Autodesk Inventor part; units mm, degrees
ref_plane "YZ Plane" through (0, 0, 0) normal (1, 0, 0) x (0, 1, 0)
ref_plane "XZ Plane" through (0, 0, 0) normal (0, 1, 0) x (-1, 0, 0)
ref_plane "XY Plane" through (0, 0, 0) normal (0, 0, 1) x (1, 0, 0)
sketch "Sketch1" plane through (0, 0, 0) normal (0, 1, 0) x (-1, 0, 0)
  line L0 (0, 0) -> (0, -14)
  circle A0 centre (0, -7) radius 8.25
  circle A1 centre (0, -7) radius 10.5
  dimension "d0" = 14
  dimension "d1" = 16.5
  dimension "d2" = 21
extrude "Extrusion1" add sketch "Sketch1" along normal blind 6
sketch "Sketch2" plane through (0, 6, -7) normal (0, 1, 0) x (1, 0, 0)
  line L0 (10.5, -10.5) -> (-10.5, -10.5)
  line L1 (-10.5, -10.5) -> (-10.5, 10.5)
  line L2 (-10.5, 10.5) -> (10.5, 10.5)
  line L3 (10.5, 10.5) -> (10.5, -10.5)
  line L4 (10.5, -10.5) -> (-10.5, 10.5) construction
  line L5 (-10.5, -10.5) -> (10.5, 10.5) construction
  circle A0 centre (0, 0) radius 10.5
  point P0 (0, -7)
extrude "Extrusion2" add sketch "Sketch2" against normal blind 6 contours L0 A0 L3 | L0 L1 A0 | A0 L2 L3 | L1 L2 A0
sketch "Sketch4" plane through (0, 6, 0) normal (0, 1, 0) x (1, 0, 0)
  circle A0 centre (0, 7) radius 8.25
  line L0 (0, 7) -> (0, -0.25)
  line L1 (0, -0.25) -> (-3.937, -0.25)
  line L2 (3.937, -0.25) -> (-3.937, -0.25)
  point P0 (0, 0)
  dimension "d14" = 7.25
extrude "Extrusion4" add sketch "Sketch4" against normal blind 6 contours L1 L2 A0 picked at (1.9893, -0.4987)
pattern_circular "Circular Pattern2" count 6 over 360 about axis through (0, 0, -7) along (0, 1, 0) of "Extrusion4"
sketch "Sketch5" plane through (0, 6, 0) normal (0, 1, 0) x (1, 0, 0)
  line L0 (-4.3102, -0.0345) -> (-8.2472, 6.7845)
  line L1 (-6.2787, 3.375) -> (6.2787, 10.625)
  line L2 (4.3102, 14.0345) -> (8.2472, 7.2155)
  line L3 (8.2472, 6.7845) -> (4.3102, -0.0345)
  line L4 (6.2787, 3.375) -> (-6.2787, 10.625)
  line L5 (-4.3102, 14.0345) -> (-8.2472, 7.2155)
  line L6 (3.937, 14.25) -> (-3.937, 14.25)
  line L7 (0, 14.25) -> (0, -0.25)
  line L8 (3.937, -0.25) -> (-3.937, -0.25)
  circle A0 centre (0, 7) radius 9.75
  line L9 (12.5, 19.5) -> (-12.5, 19.5)
  line L10 (-12.5, 19.5) -> (-12.5, -5.5)
  line L11 (-12.5, -5.5) -> (12.5, -5.5)
  line L12 (12.5, -5.5) -> (12.5, 19.5)
  line L13 (12.5, 19.5) -> (-12.5, -5.5) construction
  line L14 (-12.5, 19.5) -> (12.5, -5.5) construction
  point P0 (0, 0)
  dimension "d20" = 19.5
  dimension "d21" = 25
  dimension "d22" = 25
extrude "Extrusion5" add sketch "Sketch5" along normal blind 20
sketch "Sketch6" plane through (0, 6, 0) normal (0, -1, 0) x (1, 0, 0)
  line L0 (-10.5, -17.5) -> (10.5, -17.5)
  line L1 (10.5, -17.5) -> (10.5, 3.5)
  line L2 (10.5, 3.5) -> (-10.5, 3.5)
  line L3 (-10.5, 3.5) -> (-10.5, -17.5)
  circle A0 centre (0, -7) radius 9.75
  line L4 (-10.5, -17.5) -> (10.5, 3.5) construction
  line L5 (10.5, -17.5) -> (-10.5, 3.5) construction
  line L6 (-12.5, -19.5) -> (12.5, -19.5)
  line L7 (12.5, -19.5) -> (12.5, 5.5)
  line L8 (12.5, 5.5) -> (-12.5, 5.5)
  line L9 (-12.5, 5.5) -> (-12.5, -19.5)
  line L10 (-12.5, -19.5) -> (12.5, 5.5) construction
  line L11 (12.5, -19.5) -> (-12.5, 5.5) construction
  point P0 (0, 0)
extrude "Extrusion6" add sketch "Sketch6" along normal blind 6 contours L9 L8 L7 L6
sketch "Sketch8" plane through (-12.5, 26, 5.5) normal (0, 0, 1) x (1, 0, 0)
  line L0 (0, 0) -> (25, 0)
  line L1 (0, 0) -> (-17.5, 0)
  line L2 (25, 0) -> (42.5, 0)
  line L3 (0, 0) -> (-17.5, 0)
  line L4 (-17.5, 0) -> (-17.5, -26)
  line L5 (-17.5, -26) -> (0, -26)
  line L6 (0, -26) -> (0, 0)
  line L7 (25, 0) -> (42.5, 0)
  line L8 (42.5, 0) -> (42.5, -26)
  line L9 (42.5, -26) -> (25, -26)
  line L10 (25, -26) -> (25, 0)
  point P0 (12.5, -26)
  dimension "d27" = 17.5
  dimension "d28" = 17.5
extrude "Extrusion7" add sketch "Sketch8" against normal blind 25
sketch "Sketch9" plane through (-30, 0, 5.5) normal (0, 0, 1) x (1, 0, 0)
  line L0 (0, 26) -> (-15, 26)
  line L1 (-15, 26) -> (-15, 0)
  line L2 (-15, 0) -> (0, 0)
  line L3 (0, 0) -> (0, 26)
  line L4 (60, 26) -> (75, 26)
  line L5 (75, 26) -> (75, 0)
  line L6 (75, 0) -> (60, 0)
  line L7 (60, 0) -> (60, 26)
  point P0 (30, 0)
  dimension "d31" = 15
  dimension "d32" = 15
extrude "Extrusion8" add sketch "Sketch9" against normal blind 61.25
sketch "Sketch10" plane through (-45, 0, 5.5) normal (-1, 0, 0) x (0, 0, 1)
  line L0 (-61.25, 0) -> (-61.25, 26)
  line L1 (-61.25, 13) -> (-35, 13)
  circle A0 centre (-48.125, 13) radius 4.125
  point P0 (-5.5, 0)
  dimension "d35" = 26.25
  dimension "d36" = 8.25
extrude "Extrusion9" cut sketch "Sketch10" against normal through all
sketch "Sketch11" plane through (0, 26, 0) normal (0, 1, 0) x (1, 0, 0)
  line L0 (30, 19.5) -> (30, 24.5)
  line L1 (30, 19.5) -> (30, 55.75)
  line L2 (30, 19.5) -> (25, 19.5)
  line L3 (25, 19.5) -> (30, 24.5)
  line L4 (-30, 19.5) -> (-30, 24.5)
  line L5 (-30, 19.5) -> (-30, 55.75)
  line L6 (-30, 19.5) -> (-25, 19.5)
  line L7 (30, 19.5) -> (-30, 19.5)
  line L8 (-25, 19.5) -> (-30, 24.5)
  point P0 (0, 0)
  dimension "d39" = 5
  dimension "d40" = 5
  dimension "d41" = 5
  dimension "d42" = 5
extrude "Extrusion10" add sketch "Sketch11" against normal blind 26
sketch "Sketch12" plane through (0, 26, 0) normal (0, 1, 0) x (1, 0, 0)
  line L0 (-45, -5.5) -> (-45, 55.75)
  line L1 (45, -5.5) -> (-45, -5.5)
  line L2 (-45, -5.5) -> (-45, 24.5)
  line L3 (-45, 24.5) -> (45, 24.5)
  line L4 (45, 24.5) -> (45, -5.5)
  point P0 (0, 0)
sketch "Sketch13" plane through (0, 26, 0) normal (0, 1, 0) x (1, 0, 0)
  line L0 (45, -5.5) -> (45, 55.75)
  line L1 (45, 24.5) -> (-45, 24.5)
  line L2 (-45, 24.5) -> (-45, 55.75)
  line L3 (-45, 55.75) -> (45, 55.75)
  line L4 (45, 55.75) -> (45, 24.5)
  point P0 (0, 0)
extrude "Extrusion11" cut sketch "Sketch13" against normal through all
sketch "Sketch15" plane through (-45, 0, 5.5) normal (-1, 0, 0) x (0, 0, 1)
  line L0 (0, 0) -> (-30, 0)
  line L1 (-30, 0) -> (-30, 26)
  line L2 (-30, 26) -> (0, 26)
  line L3 (0, 26) -> (0, 0)
  point P0 (-5.5, 0)
extrude "Extrusion13" add sketch "Sketch15" along normal blind 5
sketch "Sketch16" plane through (45, 0, 5.5) normal (1, 0, 0) x (0, 0, -1)
  line L0 (30, 26) -> (0, 26)
  line L1 (0, 26) -> (0, 0)
  line L2 (0, 0) -> (30, 0)
  line L3 (30, 0) -> (30, 26)
  point P0 (5.5, 0)
extrude "Extrusion14" add sketch "Sketch16" along normal blind 5
sketch "Sketch17" plane through (-30, 0, -24.5) normal (0, 0, -1) x (-1, 0, 0)
  line L0 (20, 26) -> (20, 0)
  line L1 (20, 13) -> (15, 13)
  line L2 (0, 26) -> (0, 0)
  circle A0 centre (9.5, 13) radius 4.625
  line L3 (-80, 0) -> (-80, 26)
  line L4 (-80, 13) -> (-75, 13)
  line L5 (-60, 0) -> (-60, 26)
  line L6 (-67.5, 13) -> (-69.5, 13)
  circle A1 centre (-69.5, 13) radius 4.625
  point P0 (-30, 0)
  dimension "d55" = 5
  dimension "d58" = 9.25
  dimension "d59" = 5
  dimension "d61" = 2
  dimension "d62" = 9.25
extrude "Extrusion15" cut sketch "Sketch17" against normal blind 25
sketch "Sketch18" plane through (0, 26, 0) normal (0, 1, 0) x (1, 0, 0)
  point P0 (0, 0)
sketch "Sketch19" plane through (0, 26, 0) normal (0, 1, 0) x (1, 0, 0)
  point P0 (0, 0)
properties part number "FretterMountTop"
Build history of the part. All positions in model axes, mm. A direction names the side the tool comes from. Coordinates: 2 decimals unless noted, no trailing zeros. Order: outer loops, then holes, each group sorted by start corner. A loop starts at its lowest first (then second) coordinate and runs counter-clockwise, first axis right, second up. Notation, with made-up numbers: (-31.75, 37.25) - (-23.75, 37.25) arc R37 cw to (-23.75, 74.25) - close; hole circle Ø11 at (39, -17.5). An arc over 180 degrees is marked (long way). Write each question's results on one line, items separated by ' | '. Start each with the question number.
Item 1: Band-saw the part on A-A on x = 0. Write the cut outline in (y, z).
Item 2: Wall check: probe 1 along Y at (x, z) = (-39.5, -17.5) (3 decimals); probe 2 along Z at (x, y) = (0, 20.25); probe 3 along X at (y, z) = (16, -7). Give the ranges that are in metal, low to high. Write a range as [from, to].
Item 3: Mould opens along X. For faces 4 (the face through (-50, 13, -10)), 5 (the face through (-1, 13, 5.5)), 6 (the face through (6.306, 3.042, -3.423)) say: released by +X, released by -X, zero draft, split by the parting line, or undercut.
Item 4: Band-saw the part on B-B on z = -2.5. State how many separate pieces and enclosed holes the cut face has, and give its area (3 significant figures).
Item 5: Flat gauge pins, fed straight in: pin 1 (10 mm diameter, centred on x = 34, z = -5.5, fed in from -Y); pin 2 (5.5 mm diameter, centred on x = 39.5, y = 13, fed in from -Z); pin 3 (5 mm diameter, centred on x = 0, y = 3, fed in from -Z). Where does each tip first touch, or does it go through?
Item 6: Band-saw the part on D-D on x = 39.5. Write the cut outline in (y, z) (3 decimals), and give its area (3 significant figures).
Item 7: Band-saw the part on C-C on y = 4.5. Write the cut outline in (x, z).
Item 8: Tool access for faces 1 (the face through (0, 13, -19.5)), 2 (the face through (-6.251, 3.042, -3.327)), 3 (the face through (-6.5, 6, -3.3)): list every direction of +Z, -Z, +X, -X, +Y, -Y with a clear straight run to the whole face (end or side of a thin tool).
Numbers:
1) outline: (0, -19.5) - (26, -19.5) - (26, -16.75) - (6, -16.75) - (6, -14.25) - (0, -14.25) - close; (0, 0.25) - (6, 0.25) - (6, 2.75) - (26, 2.75) - (26, 5.5) - (0, 5.5) - close
2) probe 1: [0, 8.375], [17.625, 26] | probe 2: [-19.5, -16.75], [2.75, 5.5] | probe 3: [-50, -43.02], [-35.98, -9.75], [9.75, 35.98], [43.02, 50]
3) face 4: released by -X | face 5: zero draft | face 6: undercut
4) separate pieces: 2 | enclosed holes: 2 | area: 2,050 mm^2
5) pin 1: y = 0 | pin 2: z = 0.5 | pin 3: z = -19.5
6) outline: (0, -24.5) - (8.375, -24.5) - (8.375, 0.5) - (17.625, 0.5) - (17.625, -24.5) - (26, -24.5) - (26, 5.5) - (0, 5.5) - close | area: 549 mm^2
7) outline: (-50, -24.5) - (-30, -24.5) - (-25, -19.5) - (25, -19.5) - (30, -24.5) - (50, -24.5) - (50, 5.5) - (-50, 5.5) - close; hole (-8.25, -7.22) - (-4.31, -14.03) arc R8.25 ccw to (-3.94, -14.25) - (3.94, -14.25) arc R8.25 ccw to (4.31, -14.03) - (8.25, -7.22) arc R8.25 ccw to (8.25, -6.78) - (4.31, 0.03) arc R8.25 ccw to (3.94, 0.25) - (-3.94, 0.25) arc R8.25 ccw to (-4.31, 0.03) - (-8.25, -6.78) arc R8.25 ccw to start
8) face 1: -Z, +Y, -Y | face 2: +Y, -Y | face 3: +Y
